Input: dimensioned drawing with shaded views. Units: mm. Origin: part minimum x, y, z. Round coordinates to 2 decimals unless told otherwise and drop trailing zeros. Order: outer loops, then holes, each group sorted by start corner. A loop starts at its lowest first (then second) coordinate and runs counter-clockwise, first axis right, second up.
Item 1: First-contact query: pin 1 (2.5 mm diameter, centred on x = 4, z = 4, fed in from -Y); pin 2 (8 mm diameter, centred on x = 20.5, z = 47, fed in from +Y). Flat tips, straight axial feed; report the tip coordinate or a pass-through.
Item 2: Cut plane C-C on x = 42. Output: boundary loops of the cut face in (y, z).
Item 3: Cut plane A-A on y = 1.6. Output: boundary loops of the cut face in (x, z), then the cut area to 3 significant figures.
Item 4: Cut plane B-B on z = 50. Output: boundary loops of the cut face in (x, y).
Item 5: Mould query, pull axis Z, two halves, no side actions, for the marked faces 1 and 2. Classes: released by +Z, released by -Z, zero draft, split by the parting line, or undercut.
Item 6: Cut plane D-D on x = 34. Output: boundary loops of the cut face in (y, z), then the cut area to 3 significant figures.
Item 7: Line query: L1, parallel to X at y = 1.45, z = 4; L2, parallel to Z at x = 4, y = 1.05; L3, parallel to Z at x = 5, y = 0.4. Output: solid intervals per line, ascending.
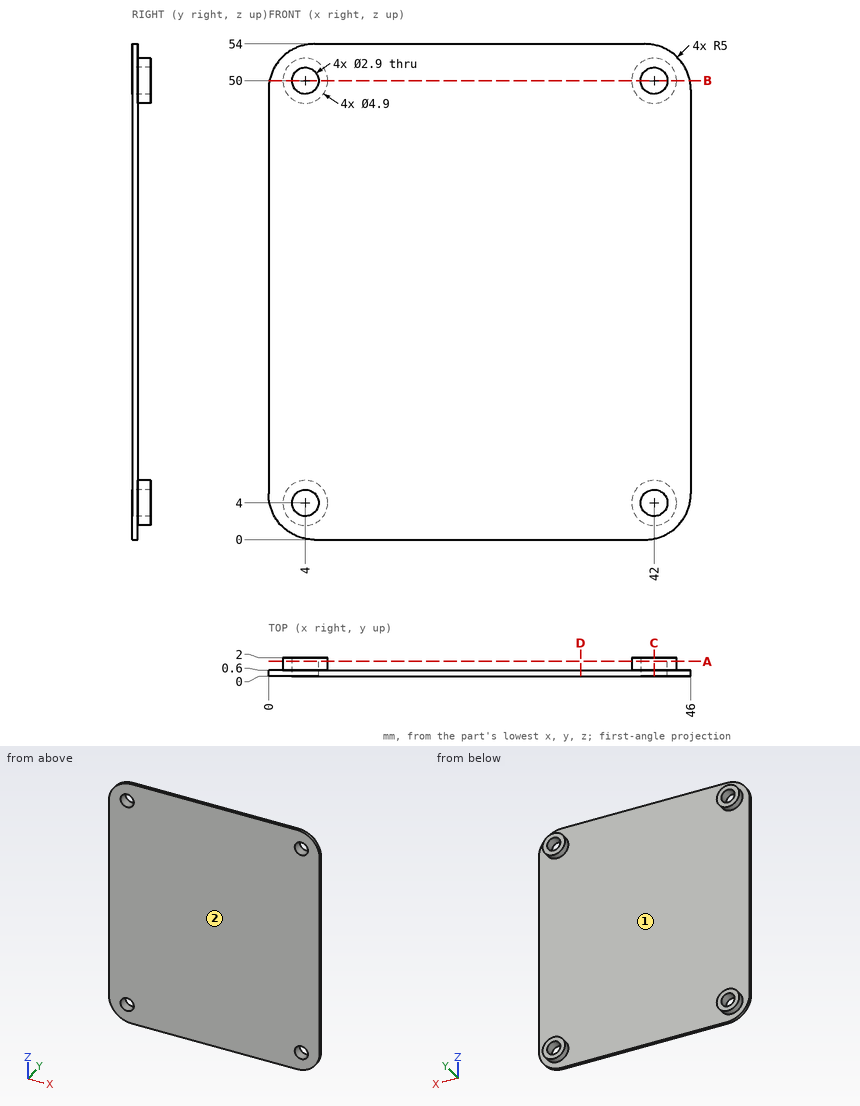
From the geometry:
1. pin 1: passes through
1. pin 2: stops at y = 0.6
2. outline: (0, 0.1) - (0.6, 0.1) - (0.6, 1.55) - (2, 1.55) - (2, 2.55) - (0, 2.55) - close; (0, 5.45) - (2, 5.45) - (2, 6.45) - (0.6, 6.45) - (0.6, 47.55) - (2, 47.55) - (2, 48.55) - (0, 48.55) - close; (0, 51.45) - (2, 51.45) - (2, 52.45) - (0.6, 52.45) - (0.6, 53.9) - (0, 53.9) - close
3. outline: circle Ø4.9 at (4, 4); circle Ø4.9 at (4, 50); circle Ø4.9 at (42, 4); circle Ø4.9 at (42, 50); hole circle Ø2.9 at (4, 4); hole circle Ø2.9 at (4, 50); hole circle Ø2.9 at (42, 4); hole circle Ø2.9 at (42, 50)
3. area: 49.0 mm2
4. outline: (0.1, 0) - (2.55, 0) - (2.55, 2) - (1.55, 2) - (1.55, 0.6) - (0.1, 0.6) - close; (5.45, 0) - (40.55, 0) - (40.55, 2) - (39.55, 2) - (39.55, 0.6) - (6.45, 0.6) - (6.45, 2) - (5.45, 2) - close; (43.45, 0) - (45.9, 0) - (45.9, 0.6) - (44.45, 0.6) - (44.45, 2) - (43.45, 2) - close
5. face 1: undercut
5. face 2: zero draft
6. outline: (0, 0) - (0.6, 0) - (0.6, 54) - (0, 54) - close
6. area: 32.4 mm2
7. L1: x = 1.55 to 2.55, 5.45 to 6.45, 39.55 to 40.55, 43.45 to 44.45
7. L2: z = 1.55 to 2.55, 5.45 to 6.45, 47.55 to 48.55, 51.45 to 52.45
7. L3: z = 0 to 2.95, 5.05 to 48.95, 51.05 to 54
